```python
from build123d import *


with BuildPart() as part:
    # Sketch1 → Revolve1 (revolve)
    with BuildSketch(Plane.XY):
        Polygon((3.5, -21.35), (12.5, -21.35), (12.5, -20.35), (6.24, -20.35), (6.24, -18.85), (12.5, -18.85), (12.5, -17.85), (6.05575, -17.85), (6.05575, -16.35), (12.5, -16.35), (12.5, -15.35), (5.8715, -15.35), (5.8715, -13.85), (12.5, -13.85), (12.5, -12.85), (5.68725, -12.85), (5.68725, -11.35), (12.5, -11.35), (12.5, -10.35), (5.503, -10.35), (5.503, -8.85), (12.5, -8.85), (12.5, -7.85), (5.31875, -7.85), (5.31875, -6.35), (12.5, -6.35), (12.5, -5.35), (5.1345, -5.35), (5.1345, -3.85), (12.5, -3.85), (12.5, -2.85), (4.95025, -2.85), (4.95025, -1.35), (12.5, -1.35), (12.5, -0.35), (4.766, -0.35), (4.766, 1.15), (12.5, 1.15), (12.5, 2.15), (4.58175, 2.15), (4.58175, 3.65), (12.5, 3.65), (12.5, 4.65), (4.3975, 4.65), (4.3975, 6.15), (12.5, 6.15), (12.5, 7.15), (4.3975, 7.15), (4.3975, 8.65), (8, 8.65), (8, 11.65), (6, 11.65), (6, 17.65), (8, 17.65), (8, 21.35), (4, 21.35), (4, 11.35), (2.1, 10.253034489), (2.1, -5.741709623), (3.5, -6.55), align=None)
    revolve(axis=Axis((0, -21.35, 0), (0, 1, 0)))


solid = part.part
```
Geometry check sheet. Reference: the model listing, model coordinates, mm. A direction names the side the tool comes from. Give positions to 0.01 mm unless a question says otherwise; leave off trailing zeros. Use a Markdown table: item, result.
Q1. Go/stop test with flat-tipped pins: P1, Ø6, axis at x = -8, z = -4, coming from the +Y side; P2, Ø10, axis at x = 9.5, y = -17, coming from the -Z side; P3, Ø12, axis at x = -8.5, y = 6.5, coming from the +Z side; P4, Ø5, axis at x = -10, y = 6, coming from the -Z side. Record where each tip stops, or that it passes through.
Computed:
| item | result |
|---|---|
| P1 | stops at y = 21.35 |
| P2 | stops at z = -11.65 |
| P3 | stops at z = 12.25 |
| P4 | stops at z = -10 |
Q2. Draft check along Y on faces 4 (the face through (-3, -21.35, 3)), 5 (the face through (2.6, -12.85, 5.4)), 6 (the face through (11.923, -0.843, -3.755)). Enter one of: pulls with the +Y half, pulls with the -Y half, needs draft (parallel to the pull), parting line crosses it, or undercut.
Computed:
| item | result |
|---|---|
| face 4 | pulls with the -Y half |
| face 5 | undercut |
| face 6 | needs draft |
Q3. Thickness scan on L1, parallel to X at y = 17.25, z = 0; L2, parallel to X at y = 5.25, z = 0. Record the ranges inside material, lowest first. Write a range as [from, to].
Computed:
| item | result |
|---|---|
| L1 | x = [-6, -4], [4, 6] |
| L2 | x = [-4.4, -2.1], [2.1, 4.4] |
Q4. Set-up check for faces 1 (the face through (11.923, 1.657, -3.755)), 2 (the face through (0, 7.15, 5)), 3 (the face through (-0.867, 16.28, 3.905)): record each of +Z, -Z, +X, -X, +Y, -Y from which the full face is reachable in a straight line by a thin tool's end or side.
Computed:
| item | result |
|---|---|
| face 1 | +Y, -Y |
| face 2 | none |
| face 3 | +Y |
Q5. Section check A-A, the plane z = -9.25. Give the number of separate pieces and of enclosed holes in the cut face, then the cut area to 3 significant figures.
Computed:
| item | result |
|---|---|
| separate pieces | 12 |
| enclosed holes | 0 |
| area | 202 mm² |
